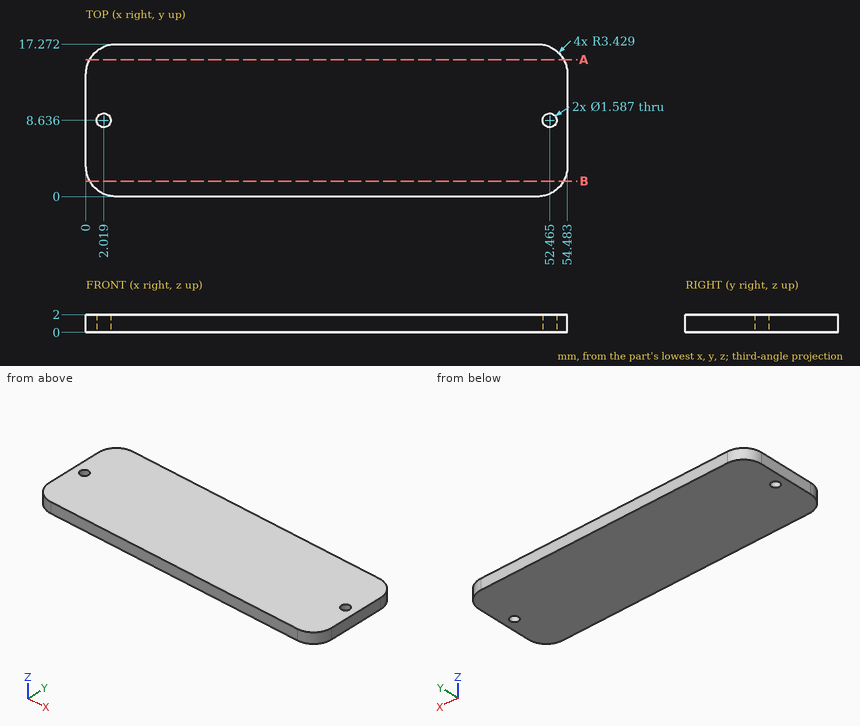
Geometry check sheet. Reference: drawing and pictorial views, mm from the part's lowest x, y, z. Give positions to 0.01 mm unless a question says otherwise; leave off trailing zeros. Order: outer loops, then holes, each group sorted by start corner. A loop starts at its lowest first (then second) coordinate and runs counter-clockwise, first axis right, second up. Notation, with made-up numbers: M 18,-13.75 L 49,-13.75 A23 ccw 49,1.25 Z; hole C -32.5,-27 d7. An arc over 180 degrees is marked long. Return JSON: item names as keys, results as strings. Group by question number.
1) Scan lines: line 1 (X direction, y = 15.75, z = 0.5) (1 decimal); line 2 (X direction, y = 14.75, z = 0.7). Record each from-to range of solid material in increasing order.
2) Section check A-A on y = 15.5. Record the cut outline in (x, z), and give its area (3 significant figures).
3) Section check B-B on y = 1.75. Record the cut outline in (x, z), and give its area (3 significant figures).
Answer block:
{
 "1": {"line 1": "x = 0.6 to 53.9", "line 2": "x = 0.12 to 54.36"},
 "2": {"outline": "M 0.43,0 L 54.06,0 L 54.06,2 L 0.43,2 Z", "area": "107 mm^2"},
 "3": {"outline": "M 0.44,0 L 54.04,0 L 54.04,2 L 0.44,2 Z", "area": "107 mm^2"}
}
